Source: CAD feature listing. Evaluate the final solid. Frame: model axes, mm. Face numbers are marked on the shaded views. Coordinates: 2 decimals unless noted, no trailing zeros. Order: outer loops, then holes, each group sorted by start corner. A loop starts at its lowest first (then second) coordinate and runs counter-clockwise, first axis right, second up.
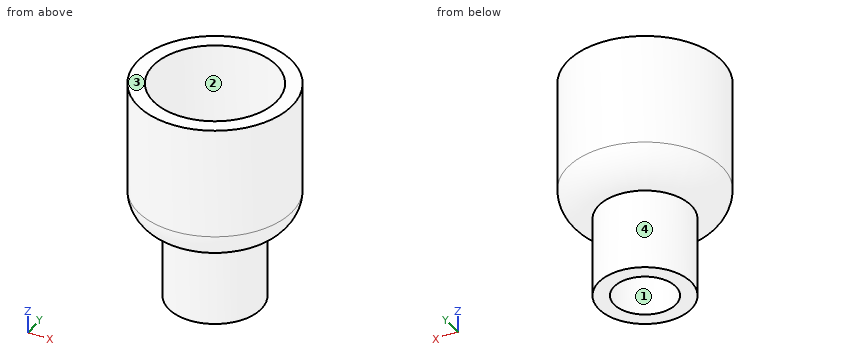
```python
from build123d import *

# Parameters (mm, degrees)
SKETCH1_R                = 7.5
BOSS_EXTRUDE1_DEPTH      = 16
BOSS_EXTRUDE2_DEPTH      = 16
BOSS_EXTRUDE2_DEPTH_BACK = 7
SKETCH2_R                = 12.5
FILLET1_R                = 5
SKETCH4_R                = 10.005
CUT_EXTRUDE1_DEPTH       = 14
SKETCH3_R                = 5.005
CUT_EXTRUDE2_DEPTH       = 10


with BuildPart() as part:
    # Sketch1 → Boss-Extrude1 (new body)
    with BuildSketch(Plane.XY):
        Circle(SKETCH1_R)
    extrude(amount=BOSS_EXTRUDE1_DEPTH)

    # Sketch2 → Boss-Extrude2 (add, two sides: drawn at the far end of the back side and taken through both)
    with BuildSketch(Plane.XY.offset(20).offset(-BOSS_EXTRUDE2_DEPTH_BACK)):
        Circle(SKETCH2_R)
    extrude(amount=BOSS_EXTRUDE2_DEPTH + BOSS_EXTRUDE2_DEPTH_BACK)

    # Fillet1
    fillet1_edges = [part.edges().sort_by_distance(p)[0] for p in [
        (-12.5, 0, 13),
    ]]
    fillet(fillet1_edges, radius=FILLET1_R - 0.0001)  # a hair under: the kernel refuses the full size

    # Sketch4 → Cut-Extrude1 (cut)
    with BuildSketch(Plane.XY.offset(36)):
        Circle(SKETCH4_R)
    extrude(amount=-CUT_EXTRUDE1_DEPTH, mode=Mode.SUBTRACT)

    # Sketch3 → Cut-Extrude2 (cut)
    with BuildSketch(Plane(origin=(0, 0, 0), x_dir=(-1, 0, 0), z_dir=(0, 0, -1))):
        Circle(SKETCH3_R)
    extrude(amount=-CUT_EXTRUDE2_DEPTH, mode=Mode.SUBTRACT)


solid = part.part
```
1. Ray query, line 1 (Y direction, x = -0.25, z = 9); line 2 (Y direction, x = 0, z = 32.25) (3 decimals); line 3 (X direction, y = -2, z = 26.5). Return the intervals inside material, ascending.
Findings:
line 1: y = -7.5 to -5, 5 to 7.5
line 2: y = -12.5 to -10.005, 10.005 to 12.5
line 3: x = -12.34 to -9.8, 9.8 to 12.34
2. Draft query along X for the marked faces 1, 2, 3 and 4. Return one class per face: released by +X, released by -X, zero draft, split by the parting line, or undercut.
Findings:
face 1: undercut
face 2: undercut
face 3: zero draft
face 4: split by the parting line
3. Section query D-D on z = 11.5. Return loops of the section in (x, y), plus the area to 3 significant figures.
Findings:
outline: circle Ø15 at (0, 0)
area: 177 mm2
4. Pin query (flat end, axial travel): P1, Ø6, axis at x = -6, z = 13.5, coming from the -Y side; P2, Ø6, axis at x = 0, y = 0, coming from the +Z side; P3, Ø5, axis at x = -8, z = 9, coming from the +Y side. Return the tip coordinate at first contact, or that it passes through.
Findings:
P1: stops at y = -11.28
P2: stops at z = 22
P3: stops at y = 5.1
5. Section query A-A on z = 27. Return loops of the section in (x, y) (3 decimals).
Findings:
outline: circle Ø25 at (0, 0); hole circle Ø20.01 at (0, 0)
